Job drawing, mm, ordinate dimensions from the low corner. One solid piece. Give positions to 0.01 mm unless a question says otherwise; leave off trailing zeros. Write each loop counter-clockwise with the first axis right and the second up, starting at its lowest first coordinate (ties: lowest second). Pieces come first, ordered by that corner, then holes. Notation, with made-up numbers: (6.5, 29) -> (14.5, 29) arc R15 ccw to (14.5, 52) -> close; hole circle Ø5 at (12, -30.5). An arc over 180 degrees is marked (long way). One line per question, with ' | ' between items. Start each with the question number.
(1) Drill centre lines: probe 1 along Y at (x, z) = (7, 5.75) (1 decimal); probe 2 along Y at (x, z) = (9.25, 7.5) (1 decimal); probe 3 along X at (y, z) = (6.5, 13.25). Where is each one in solid material? Low to high. Write a range as from..to.
(2) Pull direction Y, two halves, no side cores. Call the marked faces 1, 2 and 3: released by +Y, released by -Y, zero draft, split by the parting line, or undercut.
(3) Band-saw the part on A-A, the plane x = 5. Give the cut face in (y, z) (1 decimal).
(4) Band-saw the part on B-B, the plane y = 10.25. Give the cut face in (x, z) (1 decimal).
(5) Band-saw the part on D-D, the plane x = 2.25. Give the cut face in (y, z), and give its area (3 significant figures).
(6) Band-saw the part on C-C, the plane z = 10.5. Give the cut face in (x, y) (1 decimal).
(7) Pin check, flat tip, straight feed: P1, Ø4, axis at y = 5, z = 10, coming from the +X side. Stop position of the tip, or through.
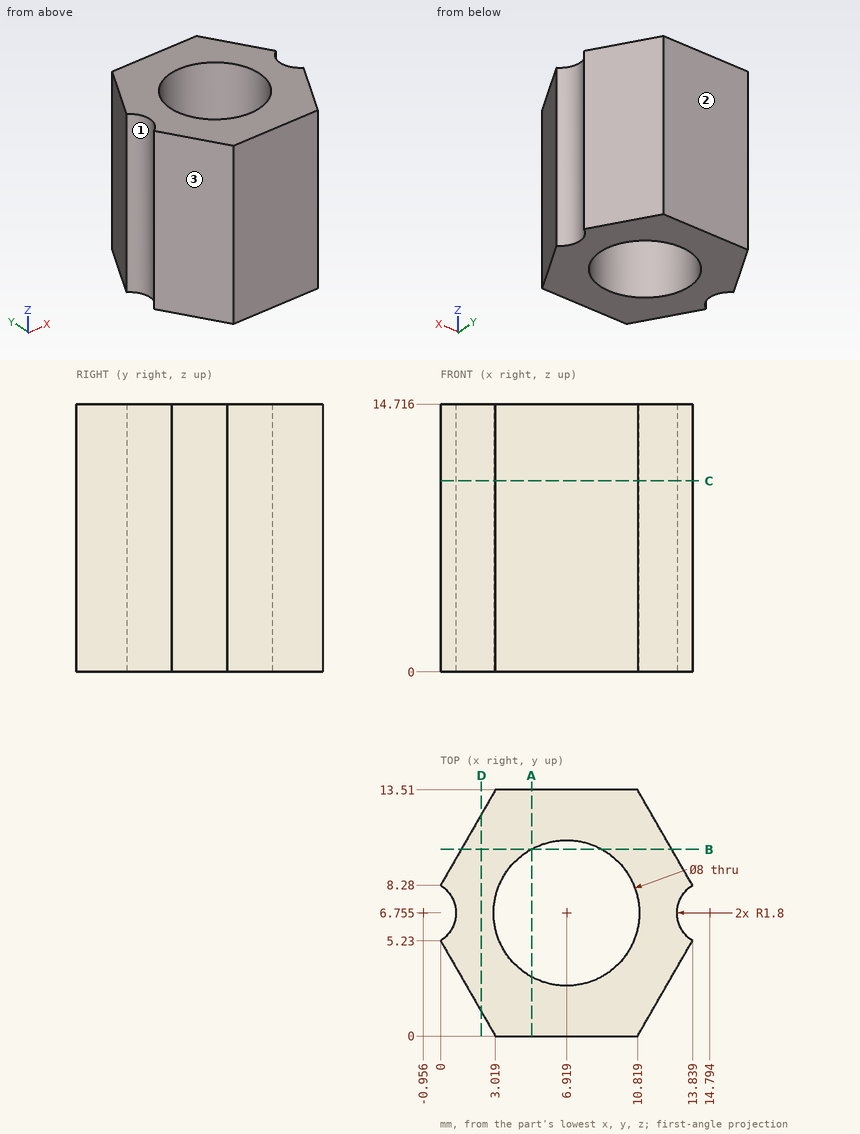
Results:
1) probe 1: y = 0..2.8, 10.8..13.5 | probe 2: y = 0..3.5, 10..13.5 | probe 3: x = 0.83..2.93, 10.91..13.01
2) face 1: undercut | face 2: released by +Y | face 3: released by -Y
3) outline: (0, 0) -> (3.2, 0) -> (3.2, 14.7) -> (0, 14.7) -> close; (10.3, 0) -> (13.5, 0) -> (13.5, 14.7) -> (10.3, 14.7) -> close
4) outline: (1.1, 0) -> (5, 0) -> (5, 14.7) -> (1.1, 14.7) -> close; (8.9, 0) -> (12.7, 0) -> (12.7, 14.7) -> (8.9, 14.7) -> close
5) outline: (1.33, 0) -> (12.18, 0) -> (12.18, 14.72) -> (1.33, 14.72) -> close | area: 160 mm²
6) outline: (0, 5.2) -> (3, 0) -> (10.8, 0) -> (13.8, 5.2) arc R1.8 cw to (13.8, 8.3) -> (10.8, 13.5) -> (3, 13.5) -> (0, 8.3) arc R1.8 cw to start; hole circle Ø8 at (6.9, 6.8)
7) P1: stops at x = 13.84
